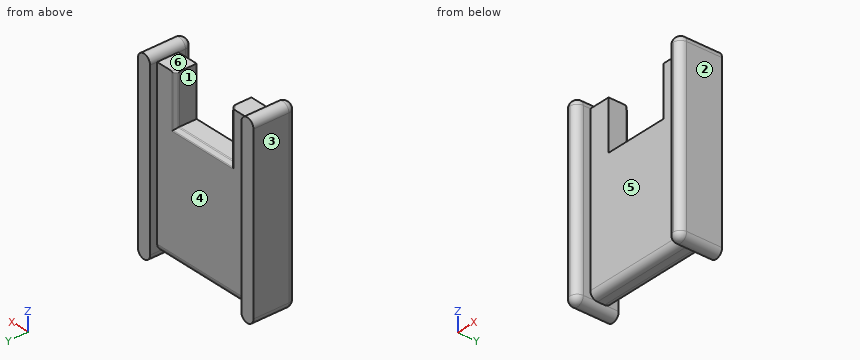
from build123d import *

# Parameters (mm, degrees)
SKETCH1_W                = 750
SKETCH1_H                = 150
BOSS_EXTRUDE1_DEPTH      = 1200
BOSS_EXTRUDE8_DEPTH      = 50
BOSS_EXTRUDE8_DEPTH_BACK = 250
FILLET2_R                = 50
FILLET3_R                = 50
SKETCH6_W                = 450
SKETCH6_H                = 350
CUT_EXTRUDE1_DEPTH       = 250
CHAMFER1_SIZE            = 25
CHAMFER2_SIZE            = 25
FILLET4_R                = 10


with BuildPart() as part:
    # Sketch1 → Boss-Extrude1 (new body)
    with BuildSketch(Plane.XY):
        with Locations((375, 75)):
            Rectangle(SKETCH1_W, SKETCH1_H)
    extrude(amount=-BOSS_EXTRUDE1_DEPTH)

    # Sketch2 → Boss-Extrude8 (add, two sides: drawn at the far end of the back side and taken through both)
    with BuildSketch(Plane(origin=(0, 150, 0), x_dir=(1, 0, 0), z_dir=(0, 1, 0)).offset(-BOSS_EXTRUDE8_DEPTH_BACK)):
        with BuildLine():
            Line((0, 1200), (0, 0))
            ThreePointArc((0, 0), (-50, -50), (-100, 0))
            Line((-100, 0), (-100, 1200))
            ThreePointArc((-100, 1200), (-50, 1250), (0, 1200))
        make_face()
        with BuildLine():
            Line((850, 1200), (850, 0))
            ThreePointArc((850, 0), (800, -50), (750, 0))
            Line((750, 0), (750, 1200))
            ThreePointArc((750, 1200), (800, 1250), (850, 1200))
        make_face()
    extrude(amount=BOSS_EXTRUDE8_DEPTH + BOSS_EXTRUDE8_DEPTH_BACK)

    # Fillet2
    fillet2_edges = [part.edges().sort_by_distance(p)[0] for p in [
        (-50, -100, -1250),
        (-100, -100, -600),
        (-50, -100, 50),
        (0, -100, -600),
        (800, -100, 50),
        (850, -100, -600),
        (800, -100, -1250),
        (750, -100, -600),
    ]]
    fillet(fillet2_edges, radius=FILLET2_R - 0.0001)  # a hair under: the kernel refuses the full size

    # Fillet3
    fillet3_edges = [part.edges().sort_by_distance(p)[0] for p in [
        (375, 150, -1200),
        (375, 0, -1200),
    ]]
    fillet(fillet3_edges, radius=FILLET3_R)

    # Sketch6 → Cut-Extrude1 (cut)
    with BuildSketch(Plane(origin=(0, 150, 0), x_dir=(1, 0, 0), z_dir=(0, 1, 0))):
        with Locations((375, 175)):
            Rectangle(SKETCH6_W, SKETCH6_H)
    extrude(amount=-CUT_EXTRUDE1_DEPTH, mode=Mode.SUBTRACT)

    # Chamfer1
    chamfer1_edges = [part.edges().sort_by_distance(p)[0] for p in [
        (375, 150, -350),
    ]]
    chamfer(chamfer1_edges, length=CHAMFER1_SIZE)

    # Chamfer2
    chamfer2_edges = [part.edges().sort_by_distance(p)[0] for p in [
        (150, 150, -187.5),
        (600, 150, -187.5),
    ]]
    chamfer(chamfer2_edges, length=CHAMFER2_SIZE)

    # Fillet4
    fillet4_edges = [part.edges().sort_by_distance(p)[0] for p in [
        (375, 125, -350),
        (375, 150, -375),
        (150, 125, -175),
        (137.5, 137.5, 0),
        (625, 150, -187.5),
        (125, 150, -187.5),
        (600, 125, -175),
        (612.5, 137.5, 0),
    ]]
    fillet(fillet4_edges, radius=FILLET4_R)


solid = part.part
Read the model definition and answer for the solid it produces. Units are mm, in the model's axes. Face numbers are marked on the shaded views. A direction names the side the tool comes from. Coordinates: 2 decimals unless noted, no trailing zeros. Write each loop counter-clockwise with the first axis right and the second up, starting at its lowest first coordinate (ties: lowest second). Pieces come first, ordered by that corner, then holes. Notation, with made-up numbers: (-2, 22) -> (44, 22) arc R19 cw to (44, 31) -> close; hole circle Ø8 at (79.25, -26.5). An arc over 180 degrees is marked (long way). Return JSON: item names as keys, results as strings.
(1) Consider line 1 along X through (y, z) = (34, -211); line 2 along X through (y, z) = (184, -753.5); line 3 along Y through (x, z) = (176, -990.5). Determine where each line is inside the solid, lowest interval first. Write a range as from..to.
Answers below:
{"line 1": "-100..150, 600..850", "line 2": "-100..0, 750..850", "line 3": "0..150"}
(2) Which of the six approach directions +Z, -Z, +X, -X, +Y, -Y give full straight-line access (tool end or side, diameter ignored) to the marked faces 4, 5 and 6?
Answers below:
{"face 4": "+Z, -Z, +Y", "face 5": "+Z, -Z, -Y", "face 6": "+Z, +Y, -Y"}
(3) The part is cut by section A-A on y = 181.5. Give the vertices of the cut face in (x, z), then the cut area to 3 significant figures.
Answers below:
{"outline": "(-100, -1200) arc R50 ccw to (0, -1200) -> (0, 0) arc R50 ccw to (-100, 0) -> close; (750, -1200) arc R50 ccw to (850, -1200) -> (850, 0) arc R50 ccw to (750, 0) -> close", "area": "256,000 mm^2"}
(4) For a pull along X with two mould halves and no side action, classify the marked faces 1, 2 and 3 as pulls with the +X half, pulls with the -X half, needs draft (parallel to the pull), parting line crosses it, or undercut.
Answers below:
{"face 1": "undercut", "face 2": "pulls with the +X half", "face 3": "pulls with the -X half"}
(5) The part is cut by section D-D on y = 70. Give the vertices of the cut face in (x, z), then the cut area to 3 significant figures.
Answers below:
{"outline": "(-100, -1200) arc R50 ccw to (0, -1200) -> (750, -1200) arc R50 ccw to (850, -1200) -> (850, 0) arc R50 ccw to (750, 0) -> (600, 0) -> (600, -350) -> (150, -350) -> (150, 0) -> (0, 0) arc R50 ccw to (-100, 0) -> close", "area": "998,000 mm^2"}
(6) The part is cut by section C-C on x = 655. Give the vertices of the cut face in (y, z), then the cut area to 3 significant figures.
Answers below:
{"outline": "(0, -1150) arc R50 ccw to (50, -1200) -> (100, -1200) arc R50 ccw to (150, -1150) -> (150, 0) -> (0, 0) -> close", "area": "179,000 mm^2"}
(7) Each of these flat-tipped pins is pushed along its axis until it touches: P1, Ø5, axis at x = 498, y = 53, coming from the +Z side; P2, Ø1.5, axis at x = 631, y = 135.5, coming from the +Z side; P3, Ø1, axis at x = 150, y = 143, coming from the +Z side. Where does it stop, or does it pass through?
Answers below:
{"P1": "z = -350", "P2": "z = 0", "P3": "z = -367.5"}
